Autodesk Fusion 360 part; units mm, degrees
sketch "Esboço1" plane through (0, 0, 0) normal (0, 0, 1) x (1, 0, 0)
  circle A0 centre (0, 0) radius 240
  circle A1 centre (148, -148) radius 5
  line L0 (-125, 204.878) -> (125, 204.878)
  circle A2 centre (0, 311.043) radius 164
  circle A3 centre (107.5, 130.5) radius 5
  line L1 (-40, 115) -> (40, 115)
  line L2 (-40, 115) -> (-40, 151.9958)
  line L3 (40, 115) -> (40, 151.9958)
  line L4 (0, 1.75) -> (0, 22.5)
  circle A4 centre (-148, -148) radius 5
  circle A5 centre (-107.5, 130.5) radius 5
  line L5 (-45, -185) -> (45, -185)
  line L6 (45, -185) -> (45, -240)
  line L7 (45, -240) -> (-45, -240)
  line L8 (-45, -240) -> (-45, -185)
  line L9 (0, -185) -> (0, -175)
  line L10 (-37.5, -175) -> (37.5, -175)
  circle A6 centre (-37.5, -175) radius 2.5
  circle A7 centre (37.5, -175) radius 2.5
  circle A8 centre (37.5, -115) radius 2.5
  circle A9 centre (37.5, -55) radius 2.5
  circle A10 centre (-37.5, -115) radius 2.5
  circle A11 centre (-37.5, -55) radius 2.5
  circle A12 centre (132.8044, 119.976) radius 2.5
  line L11 (230.3461, 81.0289) -> (182.7147, 53.5289)
  line L12 (182.7147, 53.5289) -> (137.7147, 131.4711)
  line L13 (137.7147, 131.4711) -> (185.3461, 158.9711)
  circle A13 centre (80.8429, 89.976) radius 2.5
  circle A14 centre (170.3044, 55.024) radius 2.5
  circle A15 centre (118.3429, 25.024) radius 2.5
  circle A16 centre (66.3814, -4.976) radius 2.5
  circle A17 centre (28.8814, 59.976) radius 2.5
  circle A18 centre (-170.3044, 55.024) radius 2.5
  line L14 (-185.3461, 158.9711) -> (-137.7147, 131.4711)
  line L15 (-137.7147, 131.4711) -> (-182.7147, 53.5289)
  line L16 (-182.7147, 53.5289) -> (-230.3461, 81.0289)
  circle A19 centre (-118.3429, 25.024) radius 2.5
  circle A20 centre (-132.8044, 119.976) radius 2.5
  circle A21 centre (-80.8429, 89.976) radius 2.5
  circle A22 centre (-28.8814, 59.976) radius 2.5
  circle A23 centre (-66.3814, -4.976) radius 2.5
  point P0 (0, 115)
  point P1 (0, -240)
  point P2 (-45, -235.7435)
  dimension "d1" = 480
  dimension "d13" = 10
  dimension "d14" = 148
  dimension "d15" = 148
  dimension "d16" = 250
  dimension "d17" = 328
  dimension "d18" = 10
  dimension "d19" = 130.5
  dimension "d20" = 107.5
  dimension "d21" = 115
  dimension "d22" = 80
  dimension "d25" = 90
  dimension "d26" = 55
  dimension "d27" = 10
  dimension "d28" = 75
  dimension "d29" = 5
  dimension "d30" = 5
  dimension "d33" = 1
  dimension "d34" = 60
  dimension "d36" = 360
extrude "Extrusão1" add sketch "Esboço1" along normal blind 3 contours A0 A2 L1 L2 L3 L5 L6 L8 L11 L12 L13 L14 L15 L16 | A2 L1 L2 L3
equation "d17 = ( 164 * 2 ) * 1 mm"
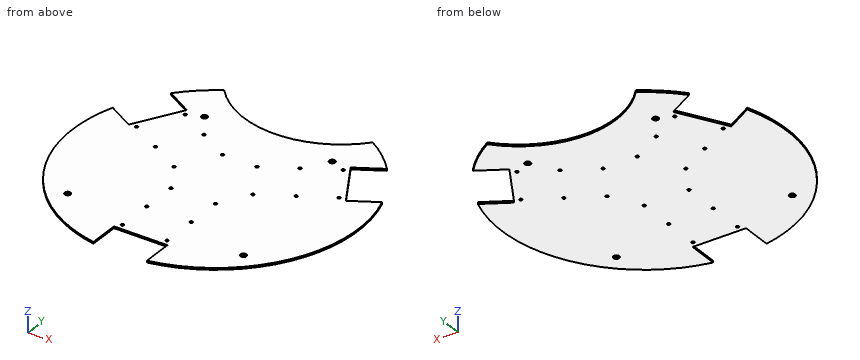
Source: CAD feature listing. Evaluate the final solid. Frame: model axes, mm. Round coordinates to 2 decimals unless told otherwise and drop trailing zeros. Write each loop counter-clockwise with the first axis right and the second up, starting at its lowest first coordinate (ties: lowest second). Pieces come first, ordered by that corner, then holes. Notation, with made-up numbers: (69.25, -3) - (97.25, -3) arc R29 ccw to (97.25, 33) - close; hole circle Ø2 at (3.25, 70.5). An arc over 180 degrees is marked (long way). Use CSV: the item, a comma, the result in double quotes. Start each with the question number.
(1) Material intervals for probe 1 along X at (y, z) = (-175, 0.85); probe 2 along Y at (x, z) = (-172.5, 0.1); probe 3 along X at (y, z) = (67.5, 2.35), sorted ascending. Write a range as [from, to].
(2) Cut plane D-D, the plane y = 44.5. Return loops of the section in (x, z), and give its area (3 significant figures).
(3) Cut plane A-A, the plane y = 163.5. Return loops of the section in (x, z).
(4) Cut plane B-B, the plane y = -133. Return loops of the section in (x, z), and give its area (3 significant figures).
(5) Cut plane C-C, the plane z = 0.65. Give the number of separate pieces and of enclosed holes in the cut face, and give its area (3 significant figures).
Geometry says:
1,probe 1,"[-164.24, -40], [-35, 35], [40, 164.24]"
1,probe 2,"[-166.86, 53.83], [56.22, 71.22], [151.55, 166.86]"
1,probe 3,"[-230.31, -206.91], [-174.65, 174.65], [206.91, 230.31]"
2,outline,"(-235.84, 0) - (235.84, 0) - (235.84, 3) - (-235.84, 3) - close"
2,area,"1,420 mm²"
3,outline,"(-175.69, 0) - (-71.6, 0) - (-71.6, 3) - (-175.69, 3) - close; (71.6, 0) - (175.69, 0) - (175.69, 3) - (71.6, 3) - close"
4,outline,"(-199.78, 0) - (199.78, 0) - (199.78, 3) - (-199.78, 3) - close"
4,area,"1,200 mm²"
5,separate pieces,"1"
5,enclosed holes,"22"
5,area,"150,000 mm²"
